Part model, mm, in its own coordinate system. A direction names the side the tool comes from. Coordinates: 2 decimals unless noted, no trailing zeros. Loops run counter-clockwise (first coordinate to the right, second up) from the corner with the lowest first, then second, coordinate; pieces in that order, holes last. Notation, with made-up numbers: (44, -29.75) - (91, -29.75) arc R33 cw to (91, 6.25) - close; hole circle Ø7 at (47, 6.25). An arc over 180 degrees is marked (long way). Use a Markdown table: item, result. Add a question column.
1) Band-saw the part on C-C (z = 22.25). Give the cut face in (x, y), plus the area to 3 significant figures.
2) Band-saw the part on B-B (y = 9). Give the cut face in (x, z).
3) Probe probe 1 along Y at (x, z) = (2.25, 28); probe 2 along Y at (x, z) = (3.25, 10.75); probe 3 along Z at (x, y) = (5.5, 9.5). List the from-to ranges inside material, lowest first. Write a range as [from, to].
4) Band-saw the part on A-A (x = 4.5). Give the cut face in (y, z), plus the area to 3 significant figures.
5) Drop flat-ended pins along their axis: P1, Ø5, axis at x = 3.5, y = 7.5, coming from the +Z side; P2, Ø2.5, axis at x = 5, z = 26, coming from the -Y side; P3, Ø0.8, axis at x = 5.5, y = 25.5, coming from the -Z side. Give the stop position or say it passes through.
6) Tool access for faces 1 (the face through (5, 25, 24)), 2 (the face through (0, 16, 17)), 3 (the face through (5, 5, 25)), 4 (the face through (10, 16, 17)), 5 (the face through (4.9, 25.5, 11.1)): list every direction of +Z, -Z, +X, -X, +Y, -Y with a clear straight run to the whole face (end or side of a thin tool).
from build123d import *

# Parameters (mm, degrees)
BOX012_W        = 10
BOX012_H        = 2
BOX012_DEPTH    = 7.8
BOX013_W        = 10
BOX013_H        = 25
BOX013_DEPTH    = 25
BOX011_W        = 10
BOX011_H        = 25
BOX011_DEPTH    = 25
CHAMFER_SIZE    = 15
CHAMFER001_SIZE = 0.4


with BuildPart() as cube011:
    # Box012 → Box012 (new body)
    with BuildSketch(Plane(origin=(0, 24, 11.1), x_dir=(1, 0, 0), z_dir=(0, 0, 1))):
        with Locations((5, 1)):
            Rectangle(BOX012_W, BOX012_H)
    extrude(amount=BOX012_DEPTH)


with BuildPart() as cube012:
    # Box013 → Box013 (new body)
    with BuildSketch(Plane(origin=(0, -14.75, 25), x_dir=(1, 0, 0), z_dir=(0, 0, 1))):
        with Locations((5, 12.5)):
            Rectangle(BOX013_W, BOX013_H)
    extrude(amount=BOX013_DEPTH)


with BuildPart() as support_profile:
    # Box011 → Box011 (new body)
    with BuildSketch(Plane.XY.offset(5)):
        with Locations((5, 12.5)):
            Rectangle(BOX011_W, BOX011_H)
    extrude(amount=BOX011_DEPTH)

    # Cut001: cut Cube012
    add(cube012.part, mode=Mode.SUBTRACT)

    # Chamfer
    chamfer_edges = [support_profile.edges().sort_by_distance(p)[0] for p in [
        (5, 0, 5),
    ]]
    chamfer(chamfer_edges, length=CHAMFER_SIZE)

    # Chamfer001
    chamfer001_edges = [support_profile.edges().sort_by_distance(p)[0] for p in [
        (5, 0, 25),
        (5, 10.25, 30),
        (5, 25, 30),
    ]]
    chamfer(chamfer001_edges, length=CHAMFER001_SIZE)

    # Fusion001002: union Cube011
    add(cube011.part)


solid = support_profile.part
Answer block:
| question | item | result |
|---|---|---|
| 1 | outline | (0, 0) - (10, 0) - (10, 25) - (0, 25) - close |
| 1 | area | 250 mm2 |
| 2 | outline | (0, 11) - (10, 11) - (10, 25) - (0, 25) - close |
| 3 | probe 1 | [10.25, 25] |
| 3 | probe 2 | [9.25, 25] |
| 3 | probe 3 | [10.5, 25] |
| 4 | outline | (0, 20) - (15, 5) - (25, 5) - (25, 11.1) - (26, 11.1) - (26, 18.9) - (25, 18.9) - (25, 29.6) - (24.6, 30) - (10.65, 30) - (10.25, 29.6) - (10.25, 25) - (0.4, 25) - (0, 24.6) - close |
| 4 | area | 469 mm2 |
| 5 | P1 | z = 25 |
| 5 | P2 | y = 0.15 |
| 5 | P3 | z = 11.1 |
| 6 | face 1 | +Z, +X, -X, +Y |
| 6 | face 2 | +Z, -Z, -X, +Y, -Y |
| 6 | face 3 | +Z, +X, -X, -Y |
| 6 | face 4 | +Z, -Z, +X, +Y, -Y |
| 6 | face 5 | -Z, +X, -X, +Y |
